Read the model definition and answer for the solid it produces. Units are mm, in the model's axes. Face numbers are marked on the shaded views. A direction names the side the tool comes from. Give positions to 0.01 mm unless a question says otherwise; leave off trailing zeros. Loops run counter-clockwise (first coordinate to the right, second up) from the corner with the lowest first, then second, coordinate; pieces in that order, holes last. Notation, with made-up numbers: (-17.75, -27.75) - (19.25, -27.75) arc R23 ccw to (19.25, 11.25) - close; hole circle Ø2 at (88, 74). An arc over 180 degrees is marked (long way). Write item = value, one per line.
Autodesk Inventor part; units mm, degrees
ref_plane "YZ Plane" through (0, 0, 0) normal (1, 0, 0) x (0, 1, 0)
ref_plane "XZ Plane" through (0, 0, 0) normal (0, 1, 0) x (-1, 0, 0)
ref_plane "XY Plane" through (0, 0, 0) normal (0, 0, 1) x (1, 0, 0)
sketch "Sketch1" plane through (0, 0, 0) normal (0, 0, 1) x (1, 0, 0)
  circle A0 centre (0, 0) radius 24
  circle A1 centre (0, 0) radius 22.6875
  dimension "d0" = 48
  dimension "d2" = 45.375
extrude "Extrusion1" add sketch "Sketch1" along normal blind 5
sketch "Sketch2" plane through (0, 0, 5) normal (0, 0, 1) x (1, 0, 0)
  circle A0 centre (0, 0) radius 24
extrude "Extrusion2" add sketch "Sketch2" along normal blind 10
sketch "Sketch3" plane through (0, 0, 0) normal (0, 0, -1) x (-1, 0, 0)
  circle A0 centre (0, 0) radius 22.6875
  circle A1 centre (0, 0) radius 24
  arc A2 (8.8161, 21.2839) -> (-8.8161, 21.2839) centre (0, 0) ccw
  arc A3 (9.0505, 21.8498) -> (-9.0505, 21.8498) centre (0, 0) ccw
  circle A4 centre (0, 0) radius 7.5
  line L0 (0, 0) -> (0, 19.001)
  line L1 (-8.8161, 21.2839) -> (-9.0505, 21.8498)
  line L2 (8.8161, 21.2839) -> (9.0505, 21.8498)
  arc A5 (-21.2839, 8.8161) -> (-21.2839, -8.8161) centre (0, 0) ccw
  arc A6 (-21.8498, 9.0505) -> (-21.8498, -9.0505) centre (0, 0) ccw
  line L3 (-21.2839, -8.8161) -> (-21.8498, -9.0505)
  line L4 (-21.2839, 8.8161) -> (-21.8498, 9.0505)
  arc A7 (-8.8161, -21.2839) -> (8.8161, -21.2839) centre (0, 0) ccw
  arc A8 (-9.0505, -21.8498) -> (9.0505, -21.8498) centre (0, 0) ccw
  line L5 (8.8161, -21.2839) -> (9.0505, -21.8498)
  line L6 (-8.8161, -21.2839) -> (-9.0505, -21.8498)
  arc A9 (21.2839, -8.8161) -> (21.2839, 8.8161) centre (0, 0) ccw
  arc A10 (21.8498, -9.0505) -> (21.8498, 9.0505) centre (0, 0) ccw
  line L7 (21.2839, 8.8161) -> (21.8498, 9.0505)
  line L8 (21.2839, -8.8161) -> (21.8498, -9.0505)
  point P0 (-19.001, 0)
  point P1 (0, -19.001)
  point P2 (19.001, 0)
  dimension "d11" = 0.35
  dimension "d10" = 0.35
  dimension "d9" = 360
ref_plane "Work Plane1" through (0, -22.4669, -8.75) normal (0, 0, -1) x (-1, 0, 0)
extrude "Extrusion6" cut sketch "Sketch3" against normal blind 10 contours A2 L1 A3 L2 | A5 L3 A6 L4 | A7 L5 A8 L6 | A9 L7 A10 L8
sketch "Sketch6" plane through (0, 0, 15) normal (0, 0, 1) x (1, 0, 0)
  circle A0 centre (0, 0) radius 7.5
  dimension "d29" = 15
extrude "Extrusion7" cut sketch "Sketch6" against normal blind 10
sketch "Sketch7" plane through (0, 0, 5) normal (0, 0, -1) x (-1, 0, 0)
  circle A0 centre (0, 0) radius 7.5493
  line L0 (-4.0263, 15.0987) -> (-4.0263, 7.5493)
  arc A1 (-4.0263, 7.5493) -> (-8.5511, -0.2878) centre (0, 0) ccw
  line L1 (-8.5511, -0.2878) -> (-15.089, -4.0625)
  arc A2 (-15.089, -4.0625) -> (-11.0627, -11.0362) centre (-13.0758, -7.5493) ccw
  line L2 (-11.0627, -11.0362) -> (-4.5248, -7.2616)
  arc A3 (-4.5248, -7.2616) -> (4.5248, -7.2616) centre (0, 0) ccw
  line L3 (4.5248, -7.2616) -> (11.0627, -11.0362)
  arc A4 (11.0627, -11.0362) -> (15.089, -4.0625) centre (13.0758, -7.5493) ccw
  line L4 (15.089, -4.0625) -> (8.5511, -0.2878)
  arc A5 (8.5511, -0.2878) -> (4.0263, 7.5493) centre (0, 0) ccw
  line L5 (4.0263, 7.5493) -> (4.0263, 15.0987)
  arc A6 (4.0263, 15.0987) -> (-4.0263, 15.0987) centre (0, 15.0987) ccw
  circle A7 centre (0, 0) radius 19.125
  circle A8 centre (0, 0) radius 7.5
  circle A9 centre (0, 0) radius 22.6875
  dimension "d34" = 38.25
extrude "Extrusion8" add sketch "Sketch7" along normal blind 2.5 contours A9
sketch "Sketch8" plane through (0, 0, 15) normal (0, 0, 1) x (1, 0, 0)
  circle A0 centre (0, 0) radius 29
  circle A1 centre (0, 0) radius 24
  dimension "d35" = 58
extrude "Extrusion9" add sketch "Sketch8" against normal up to surface (15 mm away)
sketch "Sketch9" plane through (0, 0, 0) normal (0, 0, -1) x (-1, 0, 0)
  line L0 (16.0425, 16.0425) -> (18.2743, 18.2743)
  line L1 (0, 0) -> (49.853, 0) construction
  circle A0 centre (0, 0) radius 22.6875
  circle A1 centre (0, 0) radius 29
  circle A2 centre (0, 0) radius 25.8438
  point P0 (-18.2743, 18.2743)
  point P1 (-18.2743, -18.2743)
  point P2 (18.2743, -18.2743)
  dimension "d39" = 45.375
  dimension "d41" = 51.6875
  dimension "d38" = 45
  dimension "d40" = 58
  dimension "d44" = 360
  dimension "d53" = 6.3125
hole "Hole1" at (-18.2743, 18.2743, 0) at (18.2743, 18.2743, 0) at (18.2743, -18.2743, 0) at (-18.2743, -18.2743, 0) direction (0, 0, 1) diameter 2.459 depth 8.8
sketch "Sketch10" plane through (0, 0, 0) normal (0, 0, -1) x (-1, 0, 0)
  circle A0 centre (18.2743, 18.2743) radius 1.2295
  circle A1 centre (18.2743, -18.2743) radius 1.2295
  circle A2 centre (-18.2743, -18.2743) radius 1.2295
  circle A3 centre (-18.2743, 18.2743) radius 1.2295
  point P0 (0, 0)
equation "\"d41\" = 0.5 * d40 + 0.5 * d39"
properties part number "Housing of planetary gearbox part 2" material "Steel, Alloy"
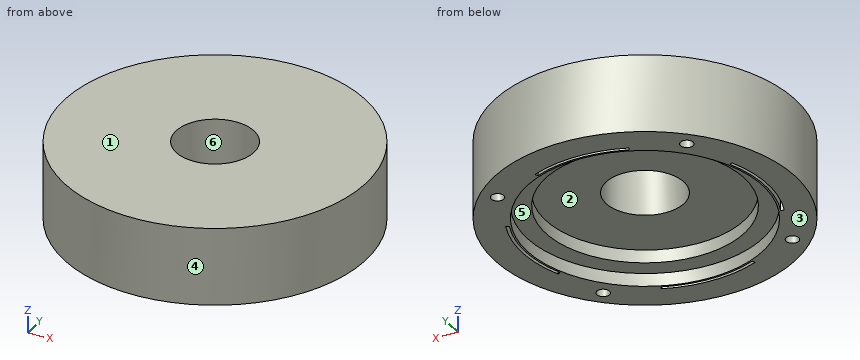
1) Find the intervals of material crossed by probe 1 along X at (y, z) = (0.5, 7.5); probe 2 along X at (y, z) = (2, 8.5); probe 3 along Y at (x, z) = (11.5, 1.75), in increasing order.
Output:
probe_1 = -29 to -23.64, -23.03 to -7.48, 7.48 to 23.03, 23.64 to 29
probe_2 = -28.93 to -23.57, -22.95 to -7.23, 7.23 to 22.95, 23.57 to 28.93
probe_3 = -26.62 to -19.56, 19.56 to 26.62
2) A cutting plane is placed at D-D on x = 10. Determine the outline of the cut face in (y, z), then the cut area to 3 significant figures.
Output:
outline = (-27.22, 0) - (-20.36, 0) - (-20.36, 2.5) - (-16.3, 2.5) - (-16.3, 5) - (16.3, 5) - (16.3, 2.5) - (20.36, 2.5) - (20.36, 0) - (27.22, 0) - (27.22, 15) - (-27.22, 15) - close
area = 633 mm²
3) A tool of negligible diameter and unlimited length cuts with its end or side. For the marked faces 1 and 2, from which of +Z, -Z, +X, -X, +Y, -Y can it reach the whole face along a straight path? Write none if from no direction.
Output:
face_1 = +Z, +X, -X, +Y, -Y
face_2 = -Z
4) The mould has two halves that part along X. Classify the marked faces 3, 4, 5 and 6: pulls with the +X half, pulls with the -X half, needs draft (parallel to the pull), parting line crosses it, or undercut.
Output:
face_3 = needs draft
face_4 = parting line crosses it
face_5 = undercut
face_6 = undercut
5) A cutting plane is placed at C-C on z = 8. Give the number of separate pieces and of enclosed holes in the cut face, then the cut area to 3 significant figures.
Output:
separate_pieces = 1
enclosed_holes = 9
area = 2,400 mm²
6) Each of these flat-tipped pins is pushed along its axis until it touches: P1, Ø5, axis at x = 9, z = 10.5, coming from the +Y side; P2, Ø1, axis at y = 7, z = 8.5, coming from the +X side; P3, Ø3, axis at y = -11.5, z = 5.5, coming from the -X side. Where does it stop, or does it pass through?
Output:
P1 = 28.26
P2 = 28.26
P3 = -27.22
